```python
from build123d import *

# Parameters (mm, degrees)
BOSS_EXTRUDE1_DEPTH = 23
SKETCH5_R           = 4
BOSS_EXTRUDE3_DEPTH = 1.7
SKETCH8_R           = 4
BOSS_EXTRUDE4_DEPTH = 1.7
SKETCH12_R          = 5.309585237
SKETCH12_R_2        = 5.383577716
SKETCH12_R_3        = 5.290961271
SKETCH12_R_4        = 5.444301549
BOSS_EXTRUDE5_DEPTH = 9.9
BOSS_EXTRUDE6_DEPTH = 22
CUT_EXTRUDE1_START  = -16
SKETCH16_R          = 11.94
CUT_EXTRUDE1_DEPTH  = 16
CUT_EXTRUDE2_START  = -16
SKETCH17_R          = 10.13
CUT_EXTRUDE2_DEPTH  = 16
CUT_EXTRUDE3_START  = -7.4
SKETCH18_R          = 5.309585237
CUT_EXTRUDE3_DEPTH  = 7.4
CUT_EXTRUDE4_START  = -7.4
SKETCH19_R          = 5.383577716
CUT_EXTRUDE4_DEPTH  = 7.4
CUT_EXTRUDE5_START  = -7.4
SKETCH20_R          = 5.444301549
CUT_EXTRUDE5_DEPTH  = 7.4
CUT_EXTRUDE6_START  = -7.4
SKETCH21_R          = 5.290961271
CUT_EXTRUDE6_DEPTH  = 7.4
SKETCH22_R          = 2.15
CUT_EXTRUDE7_DEPTH  = 10


with BuildPart() as part:
    # Sketch2 → Boss-Extrude1 (new body)
    with BuildSketch(Plane.XY):
        with BuildLine():
            Line((70.523413182, -121.258597495), (80.001788964, -115.008475165))
            ThreePointArc((80.001788964, -115.008475165), (81.651709385, -113.204688447), (82.249297777, -110.834293536))
            Line((82.249297777, -110.834293536), (82.249297777, -82.060728072))
            ThreePointArc((82.249297777, -82.060728072), (82.132627635, -80.537642087), (81.785339594, -79.050095835))
            add(Edge.make_bspline(
                [(81.785339594, -79.050095835), (81.779550585, -79.03175941), (79.763594577, -64.21980724), (72.310783114, -44.632084365), (70.089271073, -39.87053002), (68.584818962, -37.26596578)],
                knots=[0.01010668, 0.01010668, 0.01010668, 0.01010668, 0.430228508, 0.512694162, 0.834763224, 0.834763224, 0.834763224, 0.834763224], degree=3))
            ThreePointArc((68.584818962, -37.26596578), (66.377835563, -34.627803803), (63.407507036, -32.893496223))
            Line((63.407507036, -32.893496223), (39.759590264, -24.109812278))
            ThreePointArc((39.759590264, -24.109812278), (38.90305511, -23.875770322), (38.018627658, -23.796927511))
            Line((38.018627658, -23.796927511), (-39.520032104, -23.796927511))
            ThreePointArc((-39.520032104, -23.796927511), (-40.404459556, -23.875770322), (-41.26099471, -24.109812278))
            Line((-41.26099471, -24.109812278), (-64.908911482, -32.893496223))
            ThreePointArc((-64.908911482, -32.893496223), (-67.879240009, -34.627803803), (-70.086223408, -37.26596578))
            add(Edge.make_bspline(
                [(-83.28674404, -79.050095835), (-83.280955031, -79.03175941), (-81.264999023, -64.21980724), (-73.81218756, -44.632084365), (-71.590675519, -39.87053002), (-70.086223408, -37.26596578)],
                knots=[0.01010668, 0.01010668, 0.01010668, 0.01010668, 0.430228508, 0.512694162, 0.834763224, 0.834763224, 0.834763224, 0.834763224], degree=3))
            ThreePointArc((-83.28674404, -79.050095835), (-83.634032081, -80.537642087), (-83.750702223, -82.060728072))
            Line((-83.750702223, -82.060728072), (-83.750702223, -110.834293536))
            ThreePointArc((-83.750702223, -110.834293536), (-83.153113831, -113.204688447), (-81.50319341, -115.008475165))
            Line((-81.50319341, -115.008475165), (-72.024817629, -121.258597495))
            ThreePointArc((-72.024817629, -121.258597495), (-70.709179228, -121.873513284), (-69.272326442, -122.084415867))
            Line((-69.272326442, -122.084415867), (67.770921996, -122.084415867))
            ThreePointArc((67.770921996, -122.084415867), (69.207774782, -121.873513284), (70.523413182, -121.258597495))
        make_face()
    extrude(amount=BOSS_EXTRUDE1_DEPTH)

    # Sketch5 → Boss-Extrude3 (add)
    with BuildSketch(Plane.ZY.offset(83.750702223)):
        with Locations(Location((13.083649818, -90.551709518, 0), (0, 0, 90))):
            Circle(SKETCH5_R)
        with Locations(Location((13.083649818, -106.069633318, 0), (0, 0, 90))):
            Circle(SKETCH5_R)
    extrude(amount=BOSS_EXTRUDE3_DEPTH)

    # Sketch8 → Boss-Extrude4 (add)
    with BuildSketch(Plane(origin=(82.249297777, 0, 0), x_dir=(0, 0, -1), z_dir=(1, 0, 0))):
        with Locations(Location((-13.08, -90.550728072, 0), (0, 0, 270))):
            Circle(SKETCH8_R)
        with Locations(Location((-13.08, -106.070728072, 0), (0, 0, 270))):
            Circle(SKETCH8_R)
    extrude(amount=BOSS_EXTRUDE4_DEPTH)

    # Sketch12 → Boss-Extrude5 (add)
    with BuildSketch(Plane.XY.offset(23)):
        with Locations(Location((61.412858859, -56.74856372, 0), (0, 0, 180))):
            Circle(SKETCH12_R)
        with Locations(Location((61.412858859, -91.784557501, 0), (0, 0, 180))):
            Circle(SKETCH12_R_2)
        with Locations(Location((-62.293922582, -91.784557501, 0), (0, 0, 180))):
            Circle(SKETCH12_R_3)
        with Locations(Location((-62.293922582, -56.74856372, 0), (0, 0, 180))):
            Circle(SKETCH12_R_4)
        with BuildLine():
            Line((26.03317791, -39.941081705), (-26.605656617, -39.941081705))
            ThreePointArc((-26.605656617, -39.941081705), (-51.069934746, -64.405359834), (-26.605656617, -88.869637962))
            Line((-26.605656617, -88.869637962), (26.03317791, -88.869637962))
            ThreePointArc((26.03317791, -88.869637962), (50.497456038, -64.405359834), (26.03317791, -39.941081705))
        make_face()
    extrude(amount=BOSS_EXTRUDE5_DEPTH)

    # Sketch15 → Boss-Extrude6 (add)
    with BuildSketch(Plane.XY.offset(32.9)):
        with BuildLine():
            ThreePointArc((-36.30694092, -78.897586955), (-32.416918561, -54.237740907), (-7.831564022, -49.901772358))
            ThreePointArc((-7.831564022, -49.901772358), (-11.721586381, -74.561618406), (-36.30694092, -78.897586955))
        make_face()
        with BuildLine():
            ThreePointArc((33.947027157, -50.665986501), (29.727203797, -73.404384895), (7.056950152, -77.976175614))
            ThreePointArc((7.056950152, -77.976175614), (11.276773512, -55.23777722), (33.947027157, -50.665986501))
        make_face()
    extrude(amount=BOSS_EXTRUDE6_DEPTH)

    # Sketch16 → Cut-Extrude1 (cut)
    with BuildSketch(Plane.XY.offset(54.9).offset(CUT_EXTRUDE1_START)):
        with BuildLine():
            ThreePointArc((-36.30694092, -78.897586955), (-32.416918561, -54.237740907), (-7.831564022, -49.901772358))
            ThreePointArc((-7.831564022, -49.901772358), (-11.721586381, -74.561618406), (-36.30694092, -78.897586955))
        make_face()
        with Locations((-22.069252471, -64.399679657)):
            Circle(SKETCH16_R, mode=Mode.SUBTRACT)
    extrude(amount=CUT_EXTRUDE1_DEPTH, mode=Mode.SUBTRACT)

    # Sketch17 → Cut-Extrude2 (cut)
    with BuildSketch(Plane.XY.offset(54.9).offset(CUT_EXTRUDE2_START)):
        with BuildLine():
            ThreePointArc((7.056950152, -77.976175614), (11.276773512, -55.23777722), (33.947027157, -50.665986501))
            ThreePointArc((33.947027157, -50.665986501), (29.727203797, -73.404384895), (7.056950152, -77.976175614))
        make_face()
        with Locations((20.501988655, -64.321081058)):
            Circle(SKETCH17_R, mode=Mode.SUBTRACT)
    extrude(amount=CUT_EXTRUDE2_DEPTH, mode=Mode.SUBTRACT)

    # Sketch18 → Cut-Extrude3 (cut)
    with BuildSketch(Plane.XY.offset(32.9).offset(CUT_EXTRUDE3_START)):
        with Locations(Location((61.412858859, -56.74856372, 0), (0, 0, 180))):
            Circle(SKETCH18_R)
    extrude(amount=CUT_EXTRUDE3_DEPTH, mode=Mode.SUBTRACT)

    # Sketch19 → Cut-Extrude4 (cut)
    with BuildSketch(Plane.XY.offset(32.9).offset(CUT_EXTRUDE4_START)):
        with Locations(Location((61.412858859, -91.784557501, 0), (0, 0, 180))):
            Circle(SKETCH19_R)
    extrude(amount=CUT_EXTRUDE4_DEPTH, mode=Mode.SUBTRACT)

    # Sketch20 → Cut-Extrude5 (cut)
    with BuildSketch(Plane.XY.offset(32.9).offset(CUT_EXTRUDE5_START)):
        with Locations(Location((-62.293922582, -56.74856372, 0), (0, 0, 180))):
            Circle(SKETCH20_R)
    extrude(amount=CUT_EXTRUDE5_DEPTH, mode=Mode.SUBTRACT)

    # Sketch21 → Cut-Extrude6 (cut)
    with BuildSketch(Plane.XY.offset(32.9).offset(CUT_EXTRUDE6_START)):
        with Locations(Location((-62.293922582, -91.784557501, 0), (0, 0, 180))):
            Circle(SKETCH21_R)
    extrude(amount=CUT_EXTRUDE6_DEPTH, mode=Mode.SUBTRACT)

    # Sketch22 → Cut-Extrude7 (cut)
    with BuildSketch(Plane.XY.offset(25.5)):
        with Locations((-62.293922582, -56.74856372)):
            Circle(SKETCH22_R)
        with Locations((-62.293922582, -91.784557501)):
            Circle(SKETCH22_R)
        with Locations((61.412858859, -91.784557501)):
            Circle(SKETCH22_R)
        with Locations((61.412858859, -56.74856372)):
            Circle(SKETCH22_R)
    extrude(amount=-CUT_EXTRUDE7_DEPTH, mode=Mode.SUBTRACT)


solid = part.part
```
Work out the finished part from the listing and answer in its coordinate system (mm). A direction names the side the tool comes from. Round coordinates to 2 decimals unless told otherwise and drop trailing zeros. Write each loop counter-clockwise with the first axis right and the second up, starting at its lowest first coordinate (ties: lowest second). Pieces come first, ordered by that corner, then holes.
1) A cutting plane is placed at A-A on z = 30. Determine the outline of the cut face in (x, y).
2) Which of the six approach directions +Z, -Z, +X, -X, +Y, -Y give full straight-line access (tool end or side, diameter ignored) to faces 4 (the face through (82.249, -97, 11)), 5 (the face through (25.95, -55.78, 46.79)), 6 (the face through (-65, -92, 25.5))?
3) A cutting plane is placed at B-B on x = 18. Determine the outline of the cut face in (y, z).
4) Flat-ended cylindrical pins translate along their axes: P1, Ø11.5, axis at x = 64, y = -57.5, coming from the +Z side; P2, Ø5, axis at y = -62, z = 33.5, coming from the -X side; P3, Ø11, axis at x = -8, z = 29.5, coming from the -Y side. Find the tip coordinate at first contact, or state that the pin passes through.
5) Determine the mould class of faces 1 (the face through (-83.17, -113.17, 11.34)), 2 (the face through (-23.62, -52.56, 46.79)), 3 (the face through (-2, -122.084, 11)) for opening direction X: pulls with the +X half, pulls with the -X half, needs draft (parallel to the pull), parting line crosses it, or undercut.
6) Consider probe 1 along X at (y, z) = (-91, 19.5); probe 2 along Z at (x, y) = (-67, -93.5); probe 3 along Z at (x, y) = (63, -76.5). Determine where each line is inside the solid, lowest interval first.
7) A cutting plane is placed at C-C on z = 50.5. Determine the outline of the cut face in (x, y), and give its area (3 significant figures).
Entries:
1. outline: (-26.61, -88.87) - (26.03, -88.87) arc R24.46 ccw to (26.03, -39.94) - (-26.61, -39.94) arc R24.46 ccw to start
2. face 4: +X
2. face 5: +Z
2. face 6: +Z, -X, +Y, -Y
3. outline: (-122.08, 0) - (-23.8, 0) - (-23.8, 23) - (-39.94, 23) - (-39.94, 32.9) - (-50.68, 32.9) - (-50.68, 38.9) - (-54.5, 38.9) - (-54.5, 54.9) - (-74.14, 54.9) - (-74.14, 38.9) - (-79.35, 38.9) - (-79.35, 32.9) - (-88.87, 32.9) - (-88.87, 23) - (-122.08, 23) - close
4. P1: stops at z = 25.5
4. P2: stops at x = -51.07
4. P3: stops at y = -88.87
5. face 1: pulls with the -X half
5. face 2: undercut
5. face 3: needs draft
6. probe 1: x = -83.75 to -64.3, -60.29 to 59.41, 63.41 to 82.25
6. probe 2: z = 0 to 25.5
6. probe 3: z = 0 to 23
7. outline: circle Ø23.88 at (-22.07, -64.4); circle Ø20.26 at (20.5, -64.32)
7. area: 770 mm2
